```python
from build123d import *

# Parameters (mm, degrees)
EXTRUDE_1_DEPTH     = 33
SKETCH_2_W          = 113.94546963
SKETCH_2_H          = 0.153731759
SKETCH_2_W_2        = 0.159880439
SKETCH_2_H_2        = 23.946679257
CUT_EXTRUDE_1_DEPTH = 0.5
SKETCH_3_W          = 113.94546963
SKETCH_3_H          = 0.153731759
SKETCH_3_W_2        = 0.186483874
SKETCH_3_H_2        = 23.188530915
CUT_EXTRUDE_2_DEPTH = 0.5
SKETCH_4_W          = 26.780776055
SKETCH_4_H          = 92.160179523
CUT_EXTRUDE_3_DEPTH = 0.5


with BuildPart() as part:
    # 草图1 → 凸台-拉伸1 (new body)
    with BuildSketch(Plane(origin=(0, 0, 0), x_dir=(0, 0, -1), z_dir=(1, 0, 0))):
        with BuildLine():
            Line((-53, 12.5), (57, 12.5))
            ThreePointArc((57, 12.5), (58.414213562, 11.914213562), (59, 10.5))
            Line((59, 10.5), (59, -10.5))
            ThreePointArc((59, -10.5), (58.414213562, -11.914213562), (57, -12.5))
            Line((57, -12.5), (-53, -12.5))
            ThreePointArc((-53, -12.5), (-57.242640687, -10.742640687), (-59, -6.5))
            Line((-59, -6.5), (-59, 6.5))
            ThreePointArc((-59, 6.5), (-57.242640687, 10.742640687), (-53, 12.5))
        make_face()
    extrude(amount=EXTRUDE_1_DEPTH)

    # 草图2 → 切除-拉伸1 (cut)
    with BuildSketch(Plane(origin=(33, 0, 0), x_dir=(0, 0, -1), z_dir=(1, 0, 0))):
        with Locations((1.940270858, 4.299962397)):
            Rectangle(SKETCH_2_W, SKETCH_2_H)
        with Locations((1.940270858, -3.7603e-05)):
            Rectangle(SKETCH_2_W, SKETCH_2_H)
        with Locations((1.940270858, 8.599962398)):
            Rectangle(SKETCH_2_W, SKETCH_2_H)
        with Locations((1.940270858, -4.300037602)):
            Rectangle(SKETCH_2_W, SKETCH_2_H)
        with Locations((1.940270858, -8.600037603)):
            Rectangle(SKETCH_2_W, SKETCH_2_H)
        with Locations((-55.163355852, 0.001170191)):
            Rectangle(SKETCH_2_W_2, SKETCH_2_H_2)
    extrude(amount=-CUT_EXTRUDE_1_DEPTH, mode=Mode.SUBTRACT)

    # 草图3 → 切除-拉伸2 (cut)
    with BuildSketch(Plane.ZY):
        with Locations((-1.632775224, 4.336078297)):
            Rectangle(SKETCH_3_W, SKETCH_3_H)
        with Locations((-1.632775224, 0.036078297)):
            Rectangle(SKETCH_3_W, SKETCH_3_H)
        with Locations((-1.632775224, 8.636078297)):
            Rectangle(SKETCH_3_W, SKETCH_3_H)
        with Locations((-1.632775224, -4.263921704)):
            Rectangle(SKETCH_3_W, SKETCH_3_H)
        with Locations((-1.632775224, -8.563921704)):
            Rectangle(SKETCH_3_W, SKETCH_3_H)
        with Locations((55.767421869, 0.036078296)):
            Rectangle(SKETCH_3_W_2, SKETCH_3_H_2)
    extrude(amount=-CUT_EXTRUDE_2_DEPTH, mode=Mode.SUBTRACT)

    # 草图4 → 切除-拉伸3 (cut)
    with BuildSketch(Plane(origin=(0, 12.5, 0), x_dir=(1, 0, 0), z_dir=(0, 1, 0))):
        with Locations((16.455758173, 7.48146235)):
            Rectangle(SKETCH_4_W, SKETCH_4_H)
    extrude(amount=-CUT_EXTRUDE_3_DEPTH, mode=Mode.SUBTRACT)


solid = part.part
```
The listing builds one solid part. Answer for the finished solid, in the listing's coordinates (mm). Coordinates: 2 decimals unless noted, no trailing zeros. Write each loop counter-clockwise with the first axis right and the second up, starting at its lowest first coordinate (ties: lowest second). Pieces come first, ordered by that corner, then holes. Notation, with made-up numbers: (24.25, -2) - (44.25, -2) arc R18 ccw to (44.25, 21) - close; hole circle Ø7 at (49.25, 61). An arc over 180 degrees is marked (long way). One line per item, written item: value.
1) For a pull along X with two mould halves and no side action, classify faces 1 (the flat face through (16, 12, -8)), 2 (the flat face through (0, 3, -1)), 3 (the cylindrical face through (16.269, 10.696, 57.289)) as pulls with the +X half, pulls with the -X half, needs draft (parallel to the pull), parting line crosses it, or undercut.
Geometry check:
face 1: undercut
face 2: pulls with the -X half
face 3: needs draft
2) This flat-tipped pin is pushed along its axis until it touches: pin 1 Ø4 at (x, z) = (27, -15) entering from +Y. Where does it stop, or does it pass through?
Geometry check:
pin 1: stops at y = 12
3) Consider line 1 along Y through (x, z) = (19, -30); line 2 along Z through (x, y) = (27, 7); line 3 along Z through (x, y) = (5, -11.25). Determine where each line is inside the solid, lowest interval first. Write a range as from..to.
Geometry check:
line 1: y = -12.5..12
line 2: z = -59..58.98
line 3: z = -58.85..56.67
4) Find section A-A (x = 12.5). Give the vertices of the cut face in (y, z).
Geometry check:
outline: (-12.5, -57) arc R2 ccw to (-10.5, -59) - (10.5, -59) arc R2 ccw to (12.5, -57) - (12.5, -53.56) - (12, -53.56) - (12, 38.6) - (12.5, 38.6) - (12.5, 53) arc R6 ccw to (6.5, 59) - (-6.5, 59) arc R6 ccw to (-12.5, 53) - close
